Input: dimensioned drawing with shaded views. Units: mm. Origin: part minimum x, y, z. Round coordinates to 2 decimals unless told otherwise and drop trailing zeros. Loops run counter-clockwise (first coordinate to the right, second up) from the corner with the lowest first, then second, coordinate; pieces in that order, holes last.
Item 1: Section query A-A on z = 101.6. Return loops of the section in (x, y) (3 decimals).
Item 2: Section query B-B on x = 38.1. Return loops of the section in (y, z) (3 decimals).
Item 3: First-contact query: P1, Ø4, axis at x = 38.1, z = 101.6, coming from the +Y side. Flat tip, straight axial feed; report the tip coordinate or a pass-through.
Item 4: Ray query, L1, parallel to X at y = 4.75, z = 101.6 (3 decimals); L2, parallel to Z at x = 38.1, y = 8.25 (3 decimals); L3, parallel to X at y = 5, z = 102.5. Return the intervals inside material, ascending.
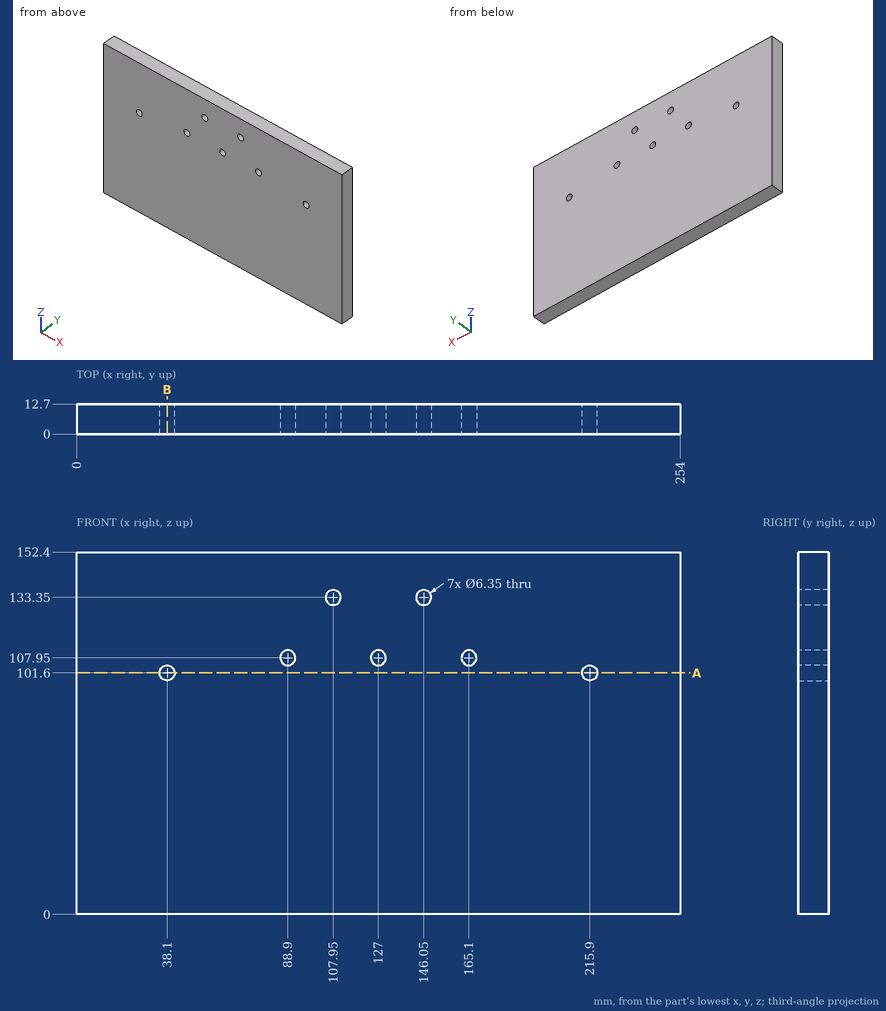
Data:
1. outline: (0, 0) - (34.925, 0) - (34.925, 12.7) - (0, 12.7) - close; (41.275, 0) - (212.725, 0) - (212.725, 12.7) - (41.275, 12.7) - close; (219.075, 0) - (254, 0) - (254, 12.7) - (219.075, 12.7) - close
2. outline: (0, 0) - (12.7, 0) - (12.7, 98.425) - (0, 98.425) - close; (0, 104.775) - (12.7, 104.775) - (12.7, 152.4) - (0, 152.4) - close
3. P1: passes through
4. L1: x = 0 to 34.925, 41.275 to 212.725, 219.075 to 254
4. L2: z = 0 to 98.425, 104.775 to 152.4
4. L3: x = 0 to 35.06, 41.14 to 212.86, 218.94 to 254
